from build123d import *

# Parameters (mm, degrees)
SKETCH1_R           = 25
SKETCH1_R_2         = 20
BOSS_EXTRUDE1_DEPTH = 3
SKETCH7_R           = 13.5
SKETCH7_R_2         = 11.1
BOSS_EXTRUDE2_DEPTH = 3
CIRPATTERN2_COUNT   = 4
SKETCH3_R           = 1.5
CUT_EXTRUDE1_DEPTH  = 4
CIRPATTERN1_COUNT   = 4


with BuildPart() as part:
    # Sketch1 → Boss-Extrude1 (new body)
    with BuildSketch(Plane.XY):
        Circle(SKETCH1_R)
        Circle(SKETCH1_R_2, mode=Mode.SUBTRACT)
    extrude(amount=BOSS_EXTRUDE1_DEPTH)



with BuildPart() as body_2:
    # Sketch7 → Boss-Extrude2 (new body)
    with BuildSketch(Plane.XY.offset(15)):
        Circle(SKETCH7_R)
        Circle(SKETCH7_R_2, mode=Mode.SUBTRACT)
    extrude(amount=BOSS_EXTRUDE2_DEPTH)


with BuildPart() as part_1:
    add(part.part)

    add(body_2.part)  # Sweep1 merges body 2
    # Sweep1: sweep along a curve in space
    with BuildLine() as sweep1_path:
        Line((0, 21.5, 3), (0, 13.5, 15))
    # Sketch8 → Sweep1 (sweep)
    with BuildSketch(Plane.XY.offset(3)):
        with BuildLine():
            Line((-4.3, 21.065611788), (-4, 19.595917942))
            ThreePointArc((-4, 19.595917942), (0, 20), (4, 19.595917942))
            Line((4, 19.595917942), (4.3, 21.065611788))
            ThreePointArc((4.3, 21.065611788), (0, 21.5), (-4.3, 21.065611788))
        make_face()
    sweep1 = sweep(path=sweep1_path.line)

    # CirPattern2: Sweep1 ×4 about axis
    cirpattern2_axis = Axis((0, 0, 0), (0, 0, -1))
    for i in range(1, CIRPATTERN2_COUNT):
        add(sweep1.rotate(cirpattern2_axis, i * 360 / CIRPATTERN2_COUNT))

    # Sketch3 → Cut-Extrude1 (cut, through all)
    with BuildSketch(Plane.XY.offset(3)):
        with Locations((15.909902577, 15.909902577)):
            Circle(SKETCH3_R)
    cut_extrude1 = extrude(amount=-CUT_EXTRUDE1_DEPTH, mode=Mode.SUBTRACT)

    # CirPattern1: Cut-Extrude1 ×4 about axis
    cirpattern1_axis = Axis((0, 0, 0), (0, 0, 1))
    for i in range(1, CIRPATTERN1_COUNT):
        add(cut_extrude1.rotate(cirpattern1_axis, i * 360 / CIRPATTERN1_COUNT), mode=Mode.SUBTRACT)


solid = part_1.part
Could you check a few things on this model? Use its own coordinates, in mm. A direction names the side the tool comes from. Coordinates: 2 decimals unless noted, no trailing zeros. Write each loop counter-clockwise with the first axis right and the second up, starting at its lowest first coordinate (ties: lowest second). Pieces come first, ordered by that corner, then holes. Notation, with made-up numbers: M -20.75,43.25 L -10.75,43.25 A22 cw -10.75,79.25 Z; hole C 87.5,-4.5 d5. An arc over 180 degrees is marked long. One line per question, with ' | ' between items.
1) Imagine slicing it at A-A, the plane y = 5. Write out the boundary of the cut face in (x, z), and give its area (3 significant figures).
Checks:
outline: M -24.49,0 L -19.36,0 L -19.36,3 L -24.49,3 Z; M -12.54,15 L -9.91,15 L -9.91,18 L -12.54,18 Z; M 9.91,15 L 12.54,15 L 12.54,18 L 9.91,18 Z; M 19.36,0 L 24.49,0 L 24.49,3 L 19.36,3 Z | area: 46.6 mm²
2) For pin 1 Ø8 at (x, z) = (1, 12.5) entering from +Y; pin 2 Ø6 at (x, z) = (17.5, 2) entering from -Y; pin 3 Ø4 at (x, y) = (5.5, 9) entering from -Z, each with a flat end and sliding along its axis, tell me the tip position at first contact or that it passes through.
Checks:
pin 1: y = 17.82 | pin 2: y = -20.37 | pin 3: z = 15
3) For faces 1 (the face through (-2.93, -13.18, 16.48)), 2 (the face through (-4.336, -19.524, 1.479)), 3 (the face through (14.8, 16.92, 1.52)), which set-ups out of +Z, -Z, +X, -X, +Y, -Y let a thin tool reach every point of the face, with its end or its side?
Checks:
face 1: +Z | face 2: -Z | face 3: +Z, -Z
4) I need wall thicknesses on probe 1 along Y at (x, z) = (0, 0.7); probe 2 along Z at (x, y) = (17, 14); probe 3 along X at (y, z) = (1, 3.5). Which ranges of each line are inside material? Lowest first, please. Write a range as [from, to].
Checks:
probe 1: [-25, -20], [20, 25] | probe 2: [0, 3] | probe 3: [-21.14, -19.64], [19.64, 21.14]
5) Imagine slicing it at B-B, the plane z = 9.25. Give the number of separate pieces and of enclosed holes in the cut face, and give its area (3 significant figures).
Checks:
separate pieces: 4 | enclosed holes: 0 | area: 50.1 mm²
